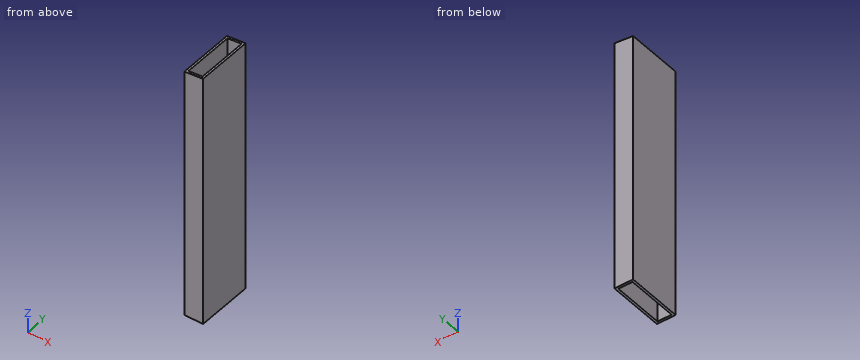
from build123d import *

# Parameters (mm, degrees)
SKETCH2_W               = 9.652
SKETCH2_H               = 3.048
SKETCH2_W_2             = 3.048
SKETCH2_H_2             = 35.052
BOSS_EXTRUDE1_DEPTH     = 343
SKETCH3_W               = 25.4
SKETCH3_H               = 76.2
SKETCH3_W_2             = 19.304
SKETCH3_H_2             = 70.104
BOSS_EXTRUDE2_DEPTH     = 50
CUT_EXTRUDE1_DEPTH      = 1
CUT_EXTRUDE1_DEPTH_BACK = 77.2


with BuildPart() as part:
    # Sketch2 → Boss-Extrude1 (new body)
    with BuildSketch(Plane.XY):
        Polygon((-12.7, 0), (-9.652, 0), (-9.652, 35.052), (-9.652, 38.1), (-12.7, 38.1), align=None)
        with Locations((-4.826, 36.576)):
            Rectangle(SKETCH2_W, SKETCH2_H)
        Polygon((0, 38.1), (0, 35.052), (9.652, 35.052), (9.652, 0), (12.7, 0), (12.7, 38.1), align=None)
        with Locations((11.176, -17.526)):
            Rectangle(SKETCH2_W_2, SKETCH2_H_2)
        Polygon((-9.652, -35.052), (-9.652, 0), (-12.7, 0), (-12.7, -38.1), (0, -38.1), (0, -35.052), align=None)
        Polygon((9.652, -35.052), (0, -35.052), (0, -38.1), (12.7, -38.1), (12.7, -35.052), align=None)
    extrude(amount=BOSS_EXTRUDE1_DEPTH)

    # Sketch3 → Boss-Extrude2 (add)
    with BuildSketch(Plane.XY.offset(343)):
        Rectangle(SKETCH3_W, SKETCH3_H)
        Rectangle(SKETCH3_W_2, SKETCH3_H_2, mode=Mode.SUBTRACT)
    extrude(amount=BOSS_EXTRUDE2_DEPTH)

    # Sketch4 → Cut-Extrude1 (cut, two sides)
    with BuildSketch(Plane(origin=(0, 38.1, 0), x_dir=(1, 0, 0), z_dir=(0, 1, 0))) as cut_extrude1_sk:
        Polygon((89.351881, -403.747167587), (94.309709366, -352.043247646), (12.7, -383.524571297), (12.7, -393), (-12.7, -393), (-12.7, -341.782211865), (-94.309709366, -333.956752354), (-99.267537732, -385.660672296), align=None)
        Polygon((12.7, -383.524571297), (94.309709366, -352.043247646), (12.7, -344.217788135), align=None)
        Polygon((12.7, -383.524571297), (12.7, -344.217788135), (0, -343), (-9.501519639, -392.088910403), align=None)
        Polygon((12.7, -393), (12.7, -383.524571297), (-9.501519639, -392.088910403), (0, -343), (-12.7, -341.782211865), (-12.7, -393), align=None)
    extrude(amount=CUT_EXTRUDE1_DEPTH, mode=Mode.SUBTRACT)
    extrude(cut_extrude1_sk.sketch, amount=-CUT_EXTRUDE1_DEPTH_BACK, mode=Mode.SUBTRACT)


solid = part.part
The model under review builds one solid part; all positions refer to its coordinate system, in mm. Give positions to 0.01 mm unless a question says otherwise; leave off trailing zeros. Loops run counter-clockwise (first coordinate to the right, second up) from the corner with the lowest first, then second, coordinate; pieces in that order, holes last. Notation, with made-up numbers: (-29, 24) -> (-21, 24) arc R24 ccw to (-21, 35) -> close; hole circle Ø5 at (70.5, 29.25). An arc over 180 degrees is marked (long way). Put each result on its own line as item: value. Start each with the question number.
1. Wall thickness on probe 1 along Y at (x, z) = (5.25, 207.5); probe 2 along X at (y, z) = (-26, 98); probe 3 along Z at (x, y) = (10.25, -30): over which ranges is each line inside the solid? List them lowest first.
2. We need section B-B on x = 0. State the section outline as (y, z) points.
3. We need section A-A on z = 241.5. State the section outline as (x, y) points, then the cut area to 3 significant figures.
4. We need section C-C on y = 11. State the section outline as (x, z) points.
5. Clearance check with a flat-ended pin moving along its axis: P1, Ø2, axis at x = -9.5, y = 10.5, coming from the +Z side. State where the tip first meets the part, or that it passes through.
Determined:
1. probe 1: -38.1 to -35.05, 35.05 to 38.1
1. probe 2: -12.7 to -9.65, 9.65 to 12.7
1. probe 3: 0 to 343.98
2. outline: (-38.1, 0) -> (-35.05, 0) -> (-35.05, 343) -> (-38.1, 343) -> close; (35.05, 0) -> (38.1, 0) -> (38.1, 343) -> (35.05, 343) -> close
3. outline: (-12.7, -38.1) -> (12.7, -38.1) -> (12.7, 38.1) -> (-12.7, 38.1) -> close; hole (-9.65, -35.05) -> (9.65, -35.05) -> (9.65, 35.05) -> (-9.65, 35.05) -> close
3. area: 582 mm^2
4. outline: (-12.7, 0) -> (-9.65, 0) -> (-9.65, 342.07) -> (-12.7, 341.78) -> close; (9.65, 0) -> (12.7, 0) -> (12.7, 344.22) -> (9.65, 343.93) -> close
5. P1: z = 342.07
